Source: CAD feature listing. Evaluate the final solid. Frame: model axes, mm. Face numbers are marked on the shaded views. A direction names the side the tool comes from. Round coordinates to 2 decimals unless told otherwise and drop trailing zeros. Write each loop counter-clockwise with the first axis right and the second up, starting at its lowest first coordinate (ties: lowest second). Pieces come first, ordered by that corner, then holes. Notation, with made-up numbers: M 0.5,70.25 L 15.5,70.25 A12 cw 15.5,75.25 Z; hole C 70.5,-3.5 d5. An arc over 180 degrees is marked long. Use a Markdown table: item, result.
```python
from build123d import *

# Parameters (mm, degrees)
F1_DEPTH = 44.45
F2_R     = 4
F3_DEPTH = 8
F4_R     = 4
F5_DEPTH = 8


with BuildPart() as f1:
    # F0 (on Top) → F1 (new body)
    with BuildSketch(Plane.XY):
        with BuildLine():
            Line((8, 44.45), (0, 44.45))
            Line((0, 44.45), (0, 8.5))
            ThreePointArc((0, 8.5), (2.489592, 2.489592), (8.5, 0))
            Line((8.5, 0), (44.45, 0))
            Line((44.45, 0), (44.45, 8))
            Line((44.45, 8), (13, 8))
            ThreePointArc((13, 8), (9.464466, 9.464466), (8, 13))
            Line((8, 13), (8, 44.45))
        make_face()
    extrude(amount=F1_DEPTH)

    # F2 (on face) → F3 (cut, through all)
    with BuildSketch(Plane.YZ.offset(8)):
        with Locations((25.4, 22.225)):
            Circle(F2_R)
    extrude(amount=-F3_DEPTH, mode=Mode.SUBTRACT)

    # F4 (on face) → F5 (cut, through all)
    with BuildSketch(Plane.XZ):
        with Locations((25.4, 22.225)):
            Circle(F4_R)
    extrude(amount=-F5_DEPTH, mode=Mode.SUBTRACT)


solid = f1.part
```
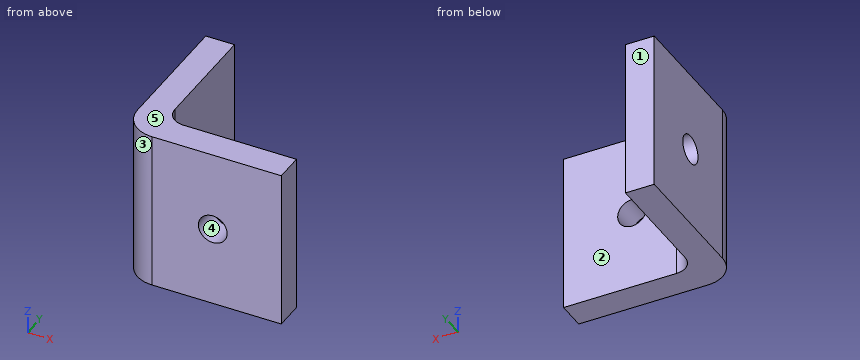
Q1. Section C-C on z = 19.5. Return loops of the section in (x, y).
Results are:
| item | result |
|---|---|
| outline | M 0,8.5 A8.5 ccw 8.5,0 L 22.47,0 L 22.47,8 L 13,8 A5 cw 8,13 L 8,22.47 L 0,22.47 Z; M 0,28.33 L 8,28.33 L 8,44.45 L 0,44.45 Z; M 28.33,0 L 44.45,0 L 44.45,8 L 28.33,8 Z |
Q2. Mould query, pull axis Z, two halves, no side actions, for the marked faces 3, 4 and 5. Classes: +Z half, -Z half, draft (parallel to the pull), parting line (faces both ways), or undercut.
Results are:
| item | result |
|---|---|
| face 3 | draft |
| face 4 | undercut |
| face 5 | +Z half |
Q3. Reachability of the marked faces 1 and 2 from +Z, -Z, +X, -X, +Y, -Y: full face, straight path, thin tool, end or side. Return the list, or none.
Results are:
| item | result |
|---|---|
| face 1 | +Z, -Z, +X, -X, +Y |
| face 2 | +Z, -Z, +X, +Y |
Q4. First-contact query: pin 1 Ø5 at (x, z) = (21.5, 16.5) entering from +Y; pin 2 Ø5 at (x, z) = (25.4, 22.225) entering from -Y; pin 3 Ø1.5 at (y, z) = (18, 5) entering from +X; pin 4 Ø6 at (y, z) = (14.5, 24) entering from +X. Flat tips, straight axial feed; report the tip coordinate or a pass-through.
Results are:
| item | result |
|---|---|
| pin 1 | y = 8 |
| pin 2 | through |
| pin 3 | x = 8 |
| pin 4 | x = 8.23 |
Q5. Line query: L1, parallel to Z at x = 6, y = 25.4 (3 decimals); L2, parallel to Y at x = 21, z = 31.5. Output: solid intervals per line, ascending.
Results are:
| item | result |
|---|---|
| L1 | 0 to 18.225, 26.225 to 44.45 |
| L2 | 0 to 8 |
Q6. Section D-D on x = 5. Return loops of the section in (y, z) (3 decimals).
Results are:
| item | result |
|---|---|
| outline | M 0.754,0 L 44.45,0 L 44.45,44.45 L 0.754,44.45 Z; hole C 25.4,22.225 d8 |
Q7. Section A-A on x = 25.4. Return loops of the section in (y, z) (3 decimals).
Results are:
| item | result |
|---|---|
| outline | M 0,0 L 8,0 L 8,18.225 L 0,18.225 Z; M 0,26.225 L 8,26.225 L 8,44.45 L 0,44.45 Z |
